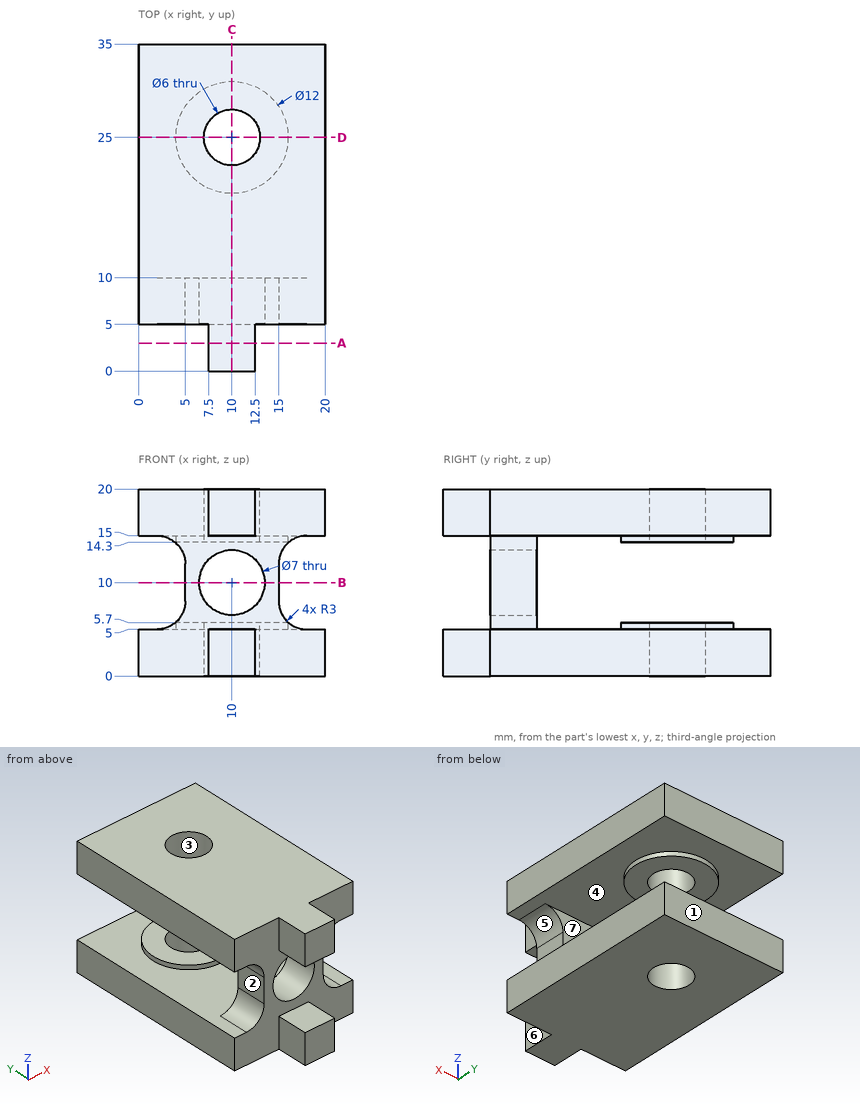
Geometry: see drawing. Coordinates: mm, zero at the bounding-box minimum. A direction names the side the tool comes from. Give positions to 0.01 mm unless a question says otherwise; leave off trailing zeros. Write each loop counter-clockwise with the first axis right and the second up, starting at its lowest first coordinate (ties: lowest second). Pieces come first, ordered by that corner, then holes. Notation, with made-up numbers: (49, 54) - (55, 54) arc R29 cw to (55, 80) - close; hole circle Ø8 at (57, 74.5). An arc over 180 degrees is marked (long way). Return JSON: item names as keys, results as strings. Group by question number.
1) Section B-B on z = 10. Return the cut outline in (x, y), plus the area to 3 significant figures.
2) Mould query, pull axis Y, two halves, no side actions, for the marked faces 1, 2 and 3. Classes: released by +Y, released by -Y, zero draft, split by the parting line, or undercut.
3) Section D-D on y = 25. Return the cut outline in (x, z), plus the area to 3 significant figures.
4) Line query: line 1 (Y direction, x = 10, z = 18.3); line 2 (Z direction, x = 5, y = 29); line 3 (Z direction, x = 10.75, y = 29). Output: solid intervals per line, ascending.
5) Section C-C on x = 10. State how many separate pieces and enclosed holes the cut face has, plus the area to 3 significant figures.
6) First-contact query: P1, Ø3, axis at y = 8.5, z = 10, coming from the -X side; P2, Ø3, axis at x = 10.5, z = 10.5, coming from the +Y side; P3, Ø1.5, axis at y = 2.5, z = 1.5, coming from the -X side; P4, Ø4.5, axis at y = 7, z = 9.5, coming from the +X side. Flat tips, straight axial feed; report the tip coordinate or a pass-through.
7) Set-up query: the marked faces 4, 5, 6 and 7. Return all of +Z, -Z, +X, -X, +Y, -Y with unobstructed straight access to the full face (end or side cutting, diameter ignored); none if empty.
8) Section A-A on y = 3. Return the cut outline in (x, z).
Filled in:
{
 "1": {"outline": "(5, 5) - (6.5, 5) - (6.5, 10) - (5, 10) - close; (13.5, 5) - (15, 5) - (15, 10) - (13.5, 10) - close", "area": "15.0 mm^2"},
 "2": {"face 1": "released by +Y", "face 2": "zero draft", "face 3": "undercut"},
 "3": {"outline": "(0, 0) - (7, 0) - (7, 5.7) - (4, 5.7) - (4, 5) - (0, 5) - close; (0, 15) - (4, 15) - (4, 14.3) - (7, 14.3) - (7, 20) - (0, 20) - close; (13, 0) - (20, 0) - (20, 5) - (16, 5) - (16, 5.7) - (13, 5.7) - close; (13, 14.3) - (16, 14.3) - (16, 15) - (20, 15) - (20, 20) - (13, 20) - close", "area": "148 mm^2"},
 "4": {"line 1": "y = 0 to 22, 28 to 35", "line 2": "z = 0 to 5, 15 to 20", "line 3": "z = 0 to 5.7, 14.3 to 20"},
 "5": {"separate pieces": "4", "enclosed holes": "0", "area": "313 mm^2"},
 "6": {"P1": "stops at x = 5", "P2": "passes through", "P3": "stops at x = 7.5", "P4": "stops at x = 15.1"},
 "7": {"face 4": "none", "face 5": "+X, +Y, -Y", "face 6": "+Z, -Z, +X, -Y", "face 7": "+X, -X"},
 "8": {"outline": "(7.5, 0) - (12.5, 0) - (12.5, 5) - (7.5, 5) - close; (7.5, 15) - (12.5, 15) - (12.5, 20) - (7.5, 20) - close"}
}
